Geometry check sheet. Reference: the model listing, model coordinates, mm. A direction names the side the tool comes from. Round coordinates to 2 decimals unless told otherwise and drop trailing zeros. Order: outer loops, then holes, each group sorted by start corner. A loop starts at its lowest first (then second) coordinate and runs counter-clockwise, first axis right, second up.
(1) Set-up check for faces 1 (the face through (-38, 23.946, 1)), 2 (the face through (-38, 31.767, 1)), 3 (the face through (-39, 28, 2.54)): record each of +Z, -Z, +X, -X, +Y, -Y from which the full face is reachable in a straight line by a thin tool's end or side.
(2) Gauge pin test, flat ends, axial feed: P1, Ø1.3, axis at x = -34.5, z = 0.5, coming from the -Y side; P2, Ø1, axis at y = 27.5, z = 1, coming from the +X side; P3, Ø1, axis at y = 31, z = 1.5, coming from the -X side. Record the tip position at first contact, or that the pin passes through.
(3) Cross-section at C-C on y = 30.25. Enter the section's corners in (x, z), and give its area (3 significant figures).
(4) Cross-section at A-A on z = 0.95. Enter the section's corners in (x, y).
(5) Cross-section at B-B on x = -33.5. Enter the section's corners in (y, z).
(6) Thickness scan on L1, parallel to Y at x = -37, z = 0.95; L2, parallel to X at y = 30.25, z = 0.4; L3, parallel to Y at x = -51, z = 2.25. Record the ranges inside material, lowest first.
from build123d import *

# Parameters (mm, degrees)
F1_DEPTH = 2.54


with BuildPart() as f1:
    # F0 (on Top) → F1 (new body)
    with BuildSketch(Plane.XY):
        with BuildLine():
            ThreePointArc((-48.2069574252, 23.9459875329), (-45.4479490063, 25.0952354669), (-44.306015985, 27.8572795006))
            ThreePointArc((-44.306015985, 27.8572795006), (-45.4187538691, 30.5897381841), (-48.123835931, 31.7674678193))
            ThreePointArc((-48.123835931, 31.7674678193), (-52.1284065306, 27.8988439109), (-48.2069574252, 23.9459875329))
        make_face()
        with BuildLine():
            ThreePointArc((-48.123835931, 31.7674678193), (-45.4187538691, 30.5897381841), (-44.306015985, 27.8572795006))
            ThreePointArc((-44.306015985, 27.8572795006), (-45.4479490063, 25.0952354669), (-48.2069574252, 23.9459875329))
            Line((-48.2069574252, 23.9459875329), (-27.4824430727, 23.9459875329))
            ThreePointArc((-27.4824430727, 23.9459875329), (-28.698975557, 25.5773806564), (-27.8223428434, 27.4139290206))
            ThreePointArc((-27.8223428434, 27.4139290206), (-28.6236525625, 28.9443668487), (-27.8413020228, 30.4845826922))
            ThreePointArc((-27.8413020228, 30.4845826922), (-28.276159726, 31.0616081435), (-28.4305025642, 31.7674678193))
            Line((-28.4305025642, 31.7674678193), (-48.123835931, 31.7674678193))
        make_face()
        with BuildLine():
            ThreePointArc((-25.048035327, 31.7674678193), (-26.7392689456, 33.4587014379), (-28.4305025642, 31.7674678193))
            ThreePointArc((-28.4305025642, 31.7674678193), (-28.276159726, 31.0616081435), (-27.8413020228, 30.4845826922))
            ThreePointArc((-27.8413020228, 30.4845826922), (-26.7392689456, 30.8404211594), (-25.6372358685, 30.4845826922))
            ThreePointArc((-25.6372358685, 30.4845826922), (-25.2023781652, 31.0616081435), (-25.048035327, 31.7674678193))
        make_face()
        with BuildLine():
            ThreePointArc((-27.8223428434, 27.4139290206), (-28.698975557, 25.5773806564), (-27.4824430727, 23.9459875329))
            ThreePointArc((-27.4824430727, 23.9459875329), (-25.6406423469, 24.1353310392), (-24.7701720222, 25.7694553584))
            ThreePointArc((-24.7701720222, 25.7694553584), (-25.0057724539, 26.7034428352), (-25.6561950478, 27.4139290206))
            ThreePointArc((-25.6561950478, 27.4139290206), (-26.7392689456, 27.0715820895), (-27.8223428434, 27.4139290206))
        make_face()
        with BuildLine():
            ThreePointArc((-25.6372358685, 30.4845826922), (-26.7392689456, 30.8404211594), (-27.8413020228, 30.4845826922))
            ThreePointArc((-27.8413020228, 30.4845826922), (-26.7392689456, 30.0762342007), (-25.6372358685, 30.4845826922))
        make_face()
        with BuildLine():
            ThreePointArc((-25.6372358685, 30.4845826922), (-26.7392689456, 30.0762342007), (-27.8413020228, 30.4845826922))
            ThreePointArc((-27.8413020228, 30.4845826922), (-28.6236525625, 28.9443668487), (-27.8223428434, 27.4139290206))
            ThreePointArc((-27.8223428434, 27.4139290206), (-26.7392689456, 27.7385522818), (-25.6561950478, 27.4139290206))
            ThreePointArc((-25.6561950478, 27.4139290206), (-25.0671441604, 28.0870737296), (-24.8548494107, 28.9560016245))
            ThreePointArc((-24.8548494107, 28.9560016245), (-25.0618111008, 29.8145889307), (-25.6372358685, 30.4845826922))
        make_face()
        with BuildLine():
            ThreePointArc((-25.6561950478, 27.4139290206), (-26.7392689456, 27.7385522818), (-27.8223428434, 27.4139290206))
            ThreePointArc((-27.8223428434, 27.4139290206), (-26.7392689456, 27.0715820895), (-25.6561950478, 27.4139290206))
        make_face()
    extrude(amount=F1_DEPTH)


solid = f1.part
Found:
1. face 1: +Z, -Z, -X, -Y
1. face 2: +Z, -Z, -X, +Y
1. face 3: +Z, +X, -X, +Y, -Y
2. P1: stops at y = 23.95
2. P2: stops at x = -25.12
2. P3: stops at x = -51.1
3. outline: (-51.31, 0) - (-25.37, 0) - (-25.37, 2.54) - (-51.31, 2.54) - close
3. area: 65.9 mm2
4. outline: (-48.21, 23.95) - (-27.48, 23.95) arc R1.97 ccw to (-25.66, 27.41) arc R1.88 ccw to (-25.64, 30.48) arc R1.69 ccw (long way) to (-28.43, 31.77) - (-48.12, 31.77) arc R3.91 ccw (long way) to start
5. outline: (23.95, 0) - (31.77, 0) - (31.77, 2.54) - (23.95, 2.54) - close
6. L1: y = 23.95 to 31.77
6. L2: x = -51.31 to -25.37
6. L3: y = 25.11 to 30.61
